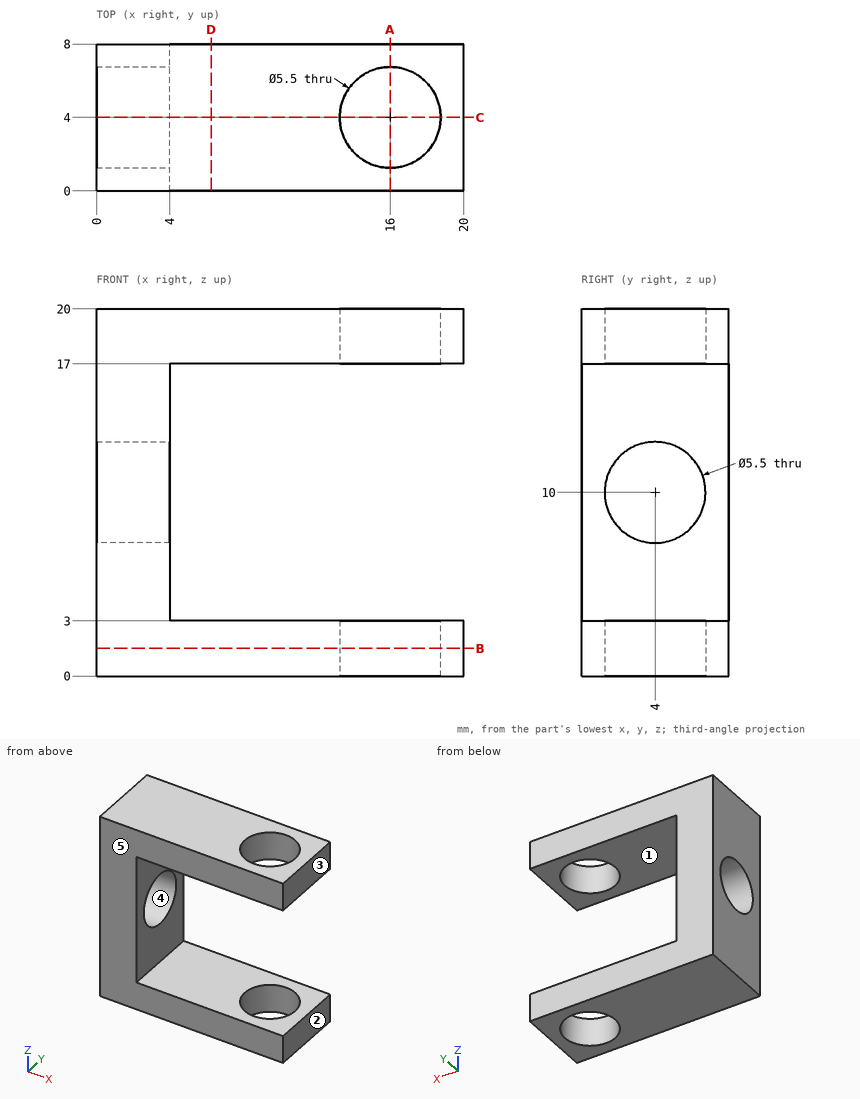
Geometry: see drawing. Coordinates: mm, zero at the bounding-box minimum. A direction names the side the tool comes from. Give positions to 0.01 mm unless a question says otherwise; leave off trailing zeros. Write each loop counter-clockwise with the first axis right and the second up, starting at its lowest first coordinate (ties: lowest second). Pieces come first, ordered by that corner, then holes. Notation, with made-up numbers: (10.5, 30) - (46.5, 30) arc R24 ccw to (46.5, 57) - close; hole circle Ø8 at (19.25, 67). An arc over 180 degrees is marked (long way). Return JSON: item names as keys, results as strings. Group by question number.
1) Section C-C on y = 4. Return the cut outline in (x, z).
2) Section B-B on z = 1.5. Return the cut outline in (x, y), plus the area to 3 significant figures.
3) Line query: line 1 (Z direction, x = 10.25, y = 3); line 2 (Y direction, x = 2.8, z = 10); line 3 (X direction, y = 4, z = 18.1). Output: solid intervals per line, ascending.
4) Section D-D on x = 6.25. Return the cut outline in (y, z), plus the area to 3 significant figures.
5) Section A-A on x = 16. Return the cut outline in (y, z).
6) Mould query, pull axis Y, two halves, no side actions, for the marked faces 3, 4 and 5. Classes: released by +Y, released by -Y, zero draft, split by the parting line, or undercut.
7) Set-up query: the marked faces 1 and 2. Return all of +Z, -Z, +X, -X, +Y, -Y with unobstructed straight access to the full face (end or side cutting, diameter ignored); none if empty.
Filled in:
{
 "1": {"outline": "(0, 0) - (13.25, 0) - (13.25, 3) - (4, 3) - (4, 7.25) - (0, 7.25) - close; (0, 12.75) - (4, 12.75) - (4, 17) - (13.25, 17) - (13.25, 20) - (0, 20) - close; (18.75, 0) - (20, 0) - (20, 3) - (18.75, 3) - close; (18.75, 17) - (20, 17) - (20, 20) - (18.75, 20) - close"},
 "2": {"outline": "(0, 0) - (20, 0) - (20, 8) - (0, 8) - close; hole circle Ø5.5 at (16, 4)", "area": "136 mm^2"},
 "3": {"line 1": "z = 0 to 3, 17 to 20", "line 2": "y = 0 to 1.25, 6.75 to 8", "line 3": "x = 0 to 13.25, 18.75 to 20"},
 "4": {"outline": "(0, 0) - (8, 0) - (8, 3) - (0, 3) - close; (0, 17) - (8, 17) - (8, 20) - (0, 20) - close", "area": "48.0 mm^2"},
 "5": {"outline": "(0, 0) - (1.25, 0) - (1.25, 3) - (0, 3) - close; (0, 17) - (1.25, 17) - (1.25, 20) - (0, 20) - close; (6.75, 0) - (8, 0) - (8, 3) - (6.75, 3) - close; (6.75, 17) - (8, 17) - (8, 20) - (6.75, 20) - close"},
 "6": {"face 3": "zero draft", "face 4": "undercut", "face 5": "released by -Y"},
 "7": {"face 1": "+X, +Y, -Y", "face 2": "+Z, -Z, +X, +Y, -Y"}
}
